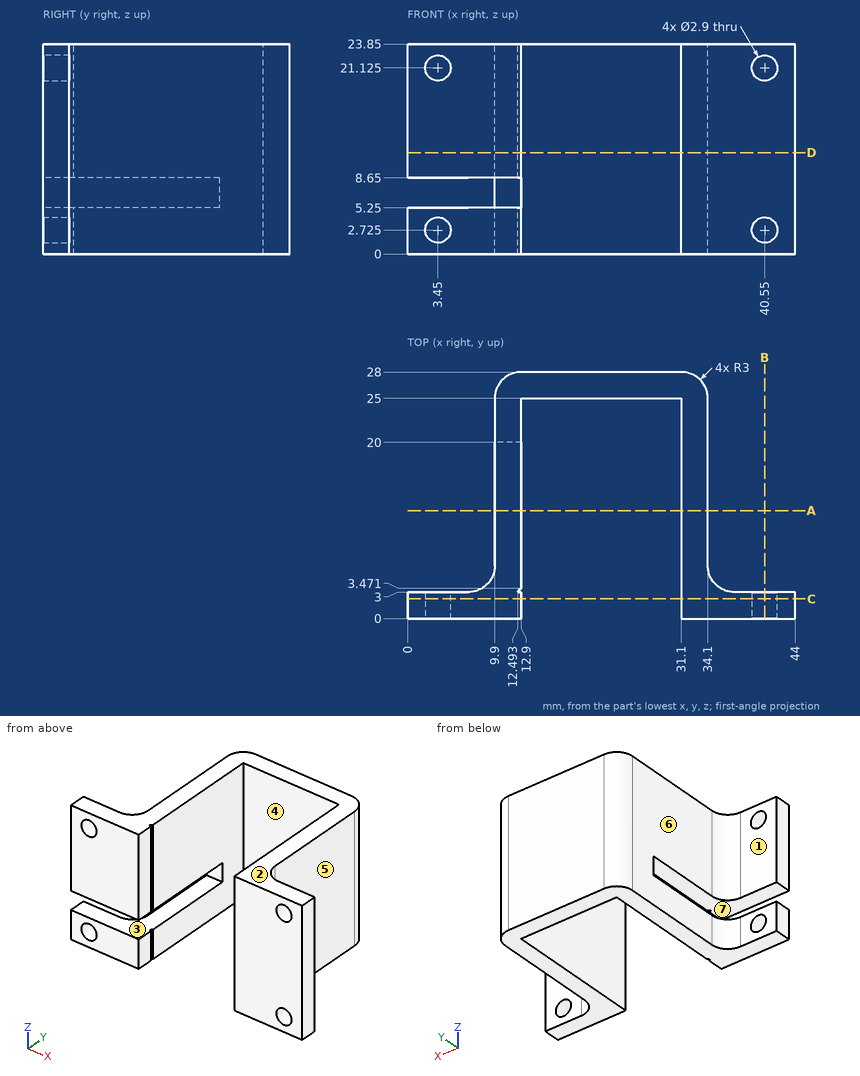
Could you check a few things on this drawing? It's one solid part, dimensions in mm from its lowest x, y, z. A direction names the side the tool comes from. Coordinates: 2 decimals unless noted, no trailing zeros. Write each loop counter-clockwise with the first axis right and the second up, starting at its lowest first coordinate (ties: lowest second). Pieces come first, ordered by that corner, then holes. Notation, with made-up numbers: (-38.5, 53) - (-17.5, 53) arc R21 cw to (-17.5, 85) - close; hole circle Ø9 at (45.5, 52.5). An arc over 180 degrees is marked (long way). Return JSON: item names as keys, results as strings. Group by question number.
Item 1: If we section it at D-D (z = 11.5): Write out the boundary of the cut face in (x, y).
Item 2: We'd pull the mould along Z, two halves only. Please class the marked faces 1, 2 and 3: pulls with the +Z half, pulls with the -Z half, needs draft (parallel to the pull), parting line crosses it, or undercut.
Item 3: If we section it at A-A (y = 12.25): Write out the boundary of the cut face in (x, z).
Item 4: Which directions (+Z, -Z, +X, -X, +Y, -Y) give clear straight access to the entire face, cutting with the end or side of a thin tool? Please do the marked faces 4, 5, 6 and 7.
Item 5: If we section it at C-C (y = 2.25): Write out the boundary of the cut face in (x, z) (3 decimals).
Item 6: Please list where these lines run through material, in increasing order: probe 1 along Z at (x, y) = (3.45, 1.65) (3 decimals); probe 2 along X at (y, z) = (22, 9); probe 3 along Y at (x, z) = (20.5, 14.75).
Item 7: If we section it at B-B (x = 40.55): Write out the boundary of the cut face in (y, z) (3 decimals).
Item 8: I'm going to push flat-ended pins straight in: pin 1 Ø7.5 at (x, z) = (40, 16) entering from +Y; pin 2 Ø12 at (y, z) = (17.5, 21) entering from -X; pin 3 Ø5.5 at (x, z) = (2.5, 19.5) entering from +Y. Where does each tip first touch, or does it pass through?
Return value:
{
 "1": {"outline": "(0, 0) - (12.9, 0) - (12.9, 3) - (12.49, 3) - (12.9, 3.47) - (12.9, 25) - (31.1, 25) - (31.1, 0) - (44, 0) - (44, 3) - (37.1, 3) arc R3 cw to (34.1, 6) - (34.1, 25) arc R3 ccw to (31.1, 28) - (12.9, 28) arc R3 ccw to (9.9, 25) - (9.9, 6) arc R3 cw to (6.9, 3) - (0, 3) - close"},
 "2": {"face 1": "needs draft", "face 2": "pulls with the +Z half", "face 3": "undercut"},
 "3": {"outline": "(9.9, 0) - (12.9, 0) - (12.9, 5.25) - (9.9, 5.25) - close; (9.9, 8.65) - (12.9, 8.65) - (12.9, 23.85) - (9.9, 23.85) - close; (31.1, 0) - (34.1, 0) - (34.1, 23.85) - (31.1, 23.85) - close"},
 "4": {"face 4": "+Z, -Z, -Y", "face 5": "+Z, -Z, +X, +Y", "face 6": "+Z, -Z, -X, +Y", "face 7": "-X, -Y"},
 "5": {"outline": "(0, 0) - (12.9, 0) - (12.9, 5.25) - (0, 5.25) - close; (0, 8.65) - (12.9, 8.65) - (12.9, 23.85) - (0, 23.85) - close; (31.1, 0) - (44, 0) - (44, 23.85) - (31.1, 23.85) - close; hole circle Ø2.9 at (3.45, 2.725); hole circle Ø2.9 at (3.45, 21.125); hole circle Ø2.9 at (40.55, 2.725); hole circle Ø2.9 at (40.55, 21.125)"},
 "6": {"probe 1": "z = 0 to 1.275, 4.175 to 5.25, 8.65 to 19.675, 22.575 to 23.85", "probe 2": "x = 9.9 to 12.9, 31.1 to 34.1", "probe 3": "y = 25 to 28"},
 "7": {"outline": "(0, 0) - (3, 0) - (3, 1.275) - (0, 1.275) - close; (0, 4.175) - (3, 4.175) - (3, 19.675) - (0, 19.675) - close; (0, 22.575) - (3, 22.575) - (3, 23.85) - (0, 23.85) - close"},
 "8": {"pin 1": "stops at y = 3.12", "pin 2": "stops at x = 9.9", "pin 3": "stops at y = 3"}
}
